Geometry: final body of the model. Coordinates: model frame, mm. A direction names the side the tool comes from. Coordinates: 2 decimals unless noted, no trailing zeros. Write each loop counter-clockwise with the first axis right and the second up, starting at its lowest first coordinate (ties: lowest second). Pieces come first, ordered by that corner, then holes. Notation, with made-up numbers: (67.5, -25.5) - (118.5, -25.5) arc R17 cw to (118.5, -14.5) - close; hole circle Ø11 at (53.5, -20.75). An arc over 180 degrees is marked (long way). Put each result on its own line as item: value.
```python
from build123d import *

# Parameters (mm, degrees)
SKETCH1_R             = 96
SKETCH1_R_2           = 88
BOSS_EXTRUDE3_DEPTH   = 208
BOSS_EXTRUDE4_DEPTH   = 60
BOSS_EXTRUDE4_2_DEPTH = 60
BOSS_EXTRUDE4_3_DEPTH = 60
BOSS_EXTRUDE4_4_DEPTH = 60
FILLET1_R             = 8
SKETCH3_R             = 2.75
CUT_EXTRUDE1_DEPTH    = 65
SKETCH5_R             = 2.75
BOSS_EXTRUDE5_DEPTH   = 20
FILLET3_R             = 5


with BuildPart() as part:
    # Sketch1 → Boss-Extrude3 (new body)
    with BuildSketch(Plane.XZ.offset(-872.688222755)):
        with Locations(Location((738.258051733, 1221.214475077, 0), (0, 0, 270))):
            Circle(SKETCH1_R)
        with Locations(Location((738.258051733, 1221.214475077, 0), (0, 0, 270))):
            Circle(SKETCH1_R_2, mode=Mode.SUBTRACT)
    extrude(amount=-BOSS_EXTRUDE3_DEPTH)


with BuildPart() as body_2:
    # Sketch2 → Boss-Extrude4 (new body)
    with BuildSketch(Plane(origin=(0, 882.688222755, 0), x_dir=(1, 0, 0), z_dir=(0, 1, 0))):
        with BuildLine():
            Line((658.258051733, -1213.714475077), (650.578236496, -1213.714475077))
            ThreePointArc((650.578236496, -1213.714475077), (650.258051733, -1221.214475077), (650.578236496, -1228.714475077))
            Line((650.578236496, -1228.714475077), (658.258051733, -1228.714475077))
            ThreePointArc((658.258051733, -1228.714475077), (665.758051733, -1221.214475077), (658.258051733, -1213.714475077))
        make_face()
    extrude(amount=BOSS_EXTRUDE4_DEPTH)


with BuildPart() as body_3:
    # Sketch2 → Boss-Extrude4 2 (new body)
    with BuildSketch(Plane(origin=(0, 882.688222755, 0), x_dir=(1, 0, 0), z_dir=(0, 1, 0))):
        with BuildLine():
            Line((730.758051733, -1301.214475077), (730.758051733, -1308.894290314))
            ThreePointArc((730.758051733, -1308.894290314), (738.258051733, -1309.214475077), (745.758051733, -1308.894290314))
            Line((745.758051733, -1308.894290314), (745.758051733, -1301.214475077))
            ThreePointArc((745.758051733, -1301.214475077), (738.258051733, -1293.714475077), (730.758051733, -1301.214475077))
        make_face()
    extrude(amount=BOSS_EXTRUDE4_2_DEPTH)


with BuildPart() as body_4:
    # Sketch2 → Boss-Extrude4 3 (new body)
    with BuildSketch(Plane(origin=(0, 882.688222755, 0), x_dir=(1, 0, 0), z_dir=(0, 1, 0))):
        with BuildLine():
            Line((818.258051733, -1228.714475077), (825.93786697, -1228.714475077))
            ThreePointArc((825.93786697, -1228.714475077), (826.258051733, -1221.214475077), (825.93786697, -1213.714475077))
            Line((825.93786697, -1213.714475077), (818.258051733, -1213.714475077))
            ThreePointArc((818.258051733, -1213.714475077), (810.758051733, -1221.214475077), (818.258051733, -1228.714475077))
        make_face()
    extrude(amount=BOSS_EXTRUDE4_3_DEPTH)


with BuildPart() as body_5:
    # Sketch2 → Boss-Extrude4 4 (new body)
    with BuildSketch(Plane(origin=(0, 882.688222755, 0), x_dir=(1, 0, 0), z_dir=(0, 1, 0))):
        with BuildLine():
            Line((730.758051733, -1141.214475077), (730.758051733, -1133.53465984))
            ThreePointArc((730.758051733, -1133.53465984), (738.258051733, -1133.214475077), (745.758051733, -1133.53465984))
            Line((745.758051733, -1133.53465984), (745.758051733, -1141.214475077))
            ThreePointArc((745.758051733, -1141.214475077), (738.258051733, -1148.714475077), (730.758051733, -1141.214475077))
        make_face()
    extrude(amount=BOSS_EXTRUDE4_4_DEPTH)

    # Combine1: union body 4, body 3, body 2, part
    add(body_4.part)
    add(body_3.part)
    add(body_2.part)
    add(part.part)

    # Fillet1
    # the kernel refuses this fillet: 8 mm, written as the material it adds along each edge
    with BuildSketch(Plane(origin=(745.758051733, 882.688222755, 1308.894290314), x_dir=(0.9902588501618923, 0, -0.13923867880745916), z_dir=(0, 1, 0)), Plane(origin=(650.578236496, 882.688222755, 1228.714475077), x_dir=(0.13923867880745078, 0, 0.9902588501618935), z_dir=(0, 1, 0)), Plane(origin=(825.93786697, 882.688222755, 1213.714475077), x_dir=(-0.13923867880746754, 0, -0.9902588501618913), z_dir=(0, 1, 0))) as fillet1_piece_1:
        with BuildLine():
            CenterArc((9.128280488, 7.988182101), FILLET1_R, 177.555452969, 95.559247246)
            Line((1.135560727, 8.329401712), (0.336288751, 8.363523673))
            ThreePointArc((0.336288751, 8.363523673), (0.277120247, 7.716395949), (-0.79220708, 0.111390943))
            Line((-0.79220708, 0.111390943), (-0.043468002, -0.79881821))
            ThreePointArc((-0.043468002, -0.79881821), (4.781480255, -0.92999689), (9.606428513, -0.79881821))
            Line((9.606428513, -0.79881821), (9.562960511, 0))
        make_face()
    extrude(amount=60)
    with BuildSketch(Plane(origin=(730.758051733, 882.688222755, 1308.894290314), x_dir=(-0.9902588501618917, 0, -0.1392386788074641), z_dir=(0, 1, 0)), Plane(origin=(650.578236496, 882.688222755, 1213.714475077), x_dir=(0.1392386788074475, 0, -0.990258850161894), z_dir=(0, 1, 0)), Plane(origin=(825.93786697, 882.688222755, 1228.714475077), x_dir=(-0.13923867880745916, 0, 0.9902588501618923), z_dir=(0, 1, 0))) as fillet1_piece_2:
        with BuildLine():
            CenterArc((9.128280488, -7.988182101), FILLET1_R, 86.885299786, 95.559247246)
            Line((1.135560727, -8.329401712), (0.336288751, -8.363523673))
            ThreePointArc((0.336288751, -8.363523673), (0.277120247, -7.716395949), (-0.79220708, -0.111390943))
            Line((-0.79220708, -0.111390943), (-0.043468002, 0.79881821))
            ThreePointArc((-0.043468002, 0.79881821), (4.781480255, 0.92999689), (9.606428513, 0.79881821))
            Line((9.606428513, 0.79881821), (9.562960511, 0))
        make_face()
    extrude(amount=60)
    with BuildSketch(Plane(origin=(745.758051733, 882.688222755, 1133.53465984), x_dir=(-0.004196280557394128, 0, 0.9999911955759828), z_dir=(0, 1, 0))) as fillet1_piece_3:
        with BuildLine():
            CenterArc((9.148032579, 7.965554461), FILLET1_R, 169.12193538, 95.559247246)
            Line((1.2917843, 9.475310394), (0.506159472, 9.626285987))
            ThreePointArc((0.506159472, 9.626285987), (-0.275580776, 4.863281082), (-0.797368322, 0.064836408))
            Line((-0.797368322, 0.064836408), (0.003357024, -0.799992956))
            ThreePointArc((0.003357024, -0.799992956), (7.683104645, -0.767766297), (8.332293668, -0.796555446))
            Line((8.332293668, -0.796555446), (8.406451751, 0))
        make_face()
    extrude(amount=60)
    with BuildSketch(Plane(origin=(730.758051733, 882.688222755, 1133.53465984), x_dir=(0.0041962805574076514, 0, 0.9999911955759828), z_dir=(0, 1, 0))) as fillet1_piece_4:
        with BuildLine():
            CenterArc((9.148032579, -7.965554461), FILLET1_R, 95.318817375, 95.559247246)
            Line((1.2917843, -9.475310394), (0.506159472, -9.626285987))
            ThreePointArc((0.506159472, -9.626285987), (-0.275580776, -4.863281082), (-0.797368322, -0.064836408))
            Line((-0.797368322, -0.064836408), (0.003357024, 0.799992956))
            ThreePointArc((0.003357024, 0.799992956), (7.683104645, 0.767766297), (8.332293668, 0.796555446))
            Line((8.332293668, 0.796555446), (8.406451751, 0))
        make_face()
    extrude(amount=60)

    # Sketch3 → Cut-Extrude1 (cut)
    with BuildSketch(Plane.XZ.offset(-882.688222755)):
        with Locations(Location((738.258051733, 1141.214475077, 0), (0, 0, 270))):
            Circle(SKETCH3_R)
        with Locations(Location((818.258051733, 1221.214475077, 0), (0, 0, 270))):
            Circle(SKETCH3_R)
        with Locations(Location((738.258051733, 1301.214475077, 0), (0, 0, 270))):
            Circle(SKETCH3_R)
        with Locations(Location((658.258051733, 1221.214475077, 0), (0, 0, 270))):
            Circle(SKETCH3_R)
    extrude(amount=-CUT_EXTRUDE1_DEPTH, mode=Mode.SUBTRACT)

    # Sketch5 → Boss-Extrude5 (add)
    # profile 1 of 4: a face of its own
    with BuildSketch(Plane(origin=(0, 1070.688222755, 0), x_dir=(1, 0, 0), z_dir=(0, 1, 0))):
        with BuildLine():
            Line((677.344338067, -1168.991103752), (671.839379876, -1163.486145561))
            ThreePointArc((671.839379876, -1163.486145561), (676.032654988, -1158.989078333), (680.529722217, -1154.79580322))
            Line((680.529722217, -1154.79580322), (686.034680408, -1160.300761412))
            ThreePointArc((686.034680408, -1160.300761412), (686.034680408, -1168.991103752), (677.344338067, -1168.991103752))
        make_face()
        with Locations(Location((681.689509238, -1164.645932582, 0), (0, 0, 270))):
            Circle(SKETCH5_R, mode=Mode.SUBTRACT)
    # profile 2 of 4: a face of its own
    with BuildSketch(Plane(origin=(0, 1070.688222755, 0), x_dir=(1, 0, 0), z_dir=(0, 1, 0))):
        with BuildLine():
            Line((677.344338068, -1273.437846402), (671.839379876, -1278.942804593))
            ThreePointArc((671.839379876, -1278.942804593), (676.032654988, -1283.439871821), (680.529722217, -1287.633146934))
            Line((680.529722217, -1287.633146934), (686.034680408, -1282.128188742))
            ThreePointArc((686.034680408, -1282.128188742), (686.034680408, -1273.437846402), (677.344338068, -1273.437846402))
        make_face()
        with Locations(Location((681.689509238, -1277.783017572, 0), (0, 0, 270))):
            Circle(SKETCH5_R, mode=Mode.SUBTRACT)
    # profile 3 of 4: a face of its own
    with BuildSketch(Plane(origin=(0, 1070.688222755, 0), x_dir=(1, 0, 0), z_dir=(0, 1, 0))):
        with BuildLine():
            Line((790.499100727, -1282.110511073), (796.005293833, -1287.616704179))
            ThreePointArc((796.005293833, -1287.616704179), (800.483448477, -1283.439871821), (804.660280835, -1278.961717178))
            Line((804.660280835, -1278.961717178), (799.154087729, -1273.455524071))
            ThreePointArc((799.154087729, -1273.455524071), (790.499100727, -1273.455524071), (790.499100727, -1282.110511073))
        make_face()
        with Locations(Location((794.826594228, -1277.783017572, 0), (0, 0, 270))):
            Circle(SKETCH5_R, mode=Mode.SUBTRACT)
    # profile 4 of 4: a face of its own
    with BuildSketch(Plane(origin=(0, 1070.688222755, 0), x_dir=(1, 0, 0), z_dir=(0, 1, 0))):
        with BuildLine():
            Line((790.499100727, -1160.318439081), (796.005293833, -1154.812245975))
            ThreePointArc((796.005293833, -1154.812245975), (800.483448477, -1158.989078333), (804.660280835, -1163.467232976))
            Line((804.660280835, -1163.467232976), (799.154087729, -1168.973426083))
            ThreePointArc((799.154087729, -1168.973426083), (790.499100727, -1168.973426083), (790.499100727, -1160.318439081))
        make_face()
        with Locations(Location((794.826594228, -1164.645932582, 0), (0, 0, 270))):
            Circle(SKETCH5_R, mode=Mode.SUBTRACT)
    extrude(amount=-BOSS_EXTRUDE5_DEPTH)

    # Fillet3
    fillet3_edges = [body_5.edges().sort_by_distance(p)[0] for p in [
        (671.839379876, 1060.688222755, 1163.486145561),
        (680.529722217, 1060.688222755, 1154.79580322),
        (680.529722217, 1060.688222755, 1287.633146934),
        (671.839379876, 1060.688222755, 1278.942804593),
        (804.660280835, 1060.688222755, 1278.961717178),
        (796.005293833, 1060.688222755, 1287.616704179),
        (796.005293833, 1060.688222755, 1154.812245975),
        (804.660280835, 1060.688222755, 1163.467232976),
    ]]
    fillet(fillet3_edges, radius=FILLET3_R)


solid = body_5.part
```
1. Ray query, probe 1 along Z at (x, y) = (738, 917); probe 2 along X at (y, z) = (923.5, 1223.5); probe 3 along X at (y, z) = (1049, 1220.5). Return the intervals inside material, ascending. Write a range as from..to.
Answer below:
probe 1: z = 1125.21..1138.48, 1143.95..1148.71, 1293.72..1298.48, 1303.95..1317.21
probe 2: x = 642.29..656.73, 659.79..665.4, 811.11..816.73, 819.79..834.23
probe 3: x = 642.26..650.26, 826.26..834.26
2. Section query B-B (x = 693). Return loops of the section in (y, z), then the cut area to 3 significant figures.
Answer below:
outline: (872.69, 1136.55) - (1080.69, 1136.55) - (1080.69, 1145.74) - (872.69, 1145.74) - close; (872.69, 1296.68) - (1080.69, 1296.68) - (1080.69, 1305.88) - (872.69, 1305.88) - close
area: 3,820 mm²
3. Section query A-A (z = 1252). Return loops of the section in (x, y).
Answer below:
outline: (647.33, 872.69) - (655.82, 872.69) - (655.82, 1080.69) - (647.33, 1080.69) - close; (820.7, 872.69) - (829.19, 872.69) - (829.19, 1080.69) - (820.7, 1080.69) - close
4. Section query D-D (y = 979). Return loops of the section in (x, z), then the cut area to 3 significant figures.
Answer below:
outline: circle Ø192 at (738.26, 1221.21); hole circle Ø176 at (738.26, 1221.21)
area: 4,620 mm²
5. Pin query (flat end, axial travel): pin 1 Ø6 at (x, y) = (767, 961) entering from +Z; pin 2 Ø8 at (y, z) = (1038, 1173.5) entering from +X; pin 3 Ø6 at (x, z) = (680, 1160) entering from +Y. Return the tip coordinate at first contact, or that it passes through.
Answer below:
pin 1: stops at z = 1313.7
pin 2: stops at x = 823.73
pin 3: stops at y = 1070.69
6. Section query C-C (x = 751). Return loops of the section in (y, z).
Answer below:
outline: (872.69, 1126.06) - (1080.69, 1126.06) - (1080.69, 1134.14) - (942.69, 1134.14) - (942.69, 1135.18) - (882.69, 1135.18) - (882.69, 1134.14) - (872.69, 1134.14) - close; (872.69, 1308.29) - (882.69, 1308.29) - (882.69, 1307.25) - (942.69, 1307.25) - (942.69, 1308.29) - (1080.69, 1308.29) - (1080.69, 1316.37) - (872.69, 1316.37) - close
7. Mould query, pull axis Z, two halves, no side actions, for faces 4 (the cylindrical face through (748.984, 912.268, 1136.243)), 5 (the cylindrical face through (767.094, 975.232, 1129.648)), 6 (the flat face through (660, 872.688, 1179)). Classes: +Z half, -Z half, draft (parallel to the pull), parting line (faces both ways), or undercut.
Answer below:
face 4: undercut
face 5: parting line
face 6: draft
8. Set-up query: faces 1 (the flat face through (822, 942.688, 1221)), 2 (the flat face through (798, 1050.688, 1279)), 3 (the cylindrical face through (748.83, 912.27, 1306.07)). Return all of +Z, -Z, +X, -X, +Y, -Y with unobstructed straight access to the full face (end or side cutting, diameter ignored); none if empty.
Answer below:
face 1: +Y
face 2: -Y
face 3: +Y, -Y
